Geometry check sheet. Reference: the model listing, model coordinates, mm. Face numbers are marked on the shaded views. Give positions to 0.01 mm unless a question says otherwise; leave off trailing zeros. Loops run counter-clockwise (first coordinate to the right, second up) from the corner with the lowest first, then second, coordinate; pieces in that order, holes last.
```python
from build123d import *

# Parameters (mm, degrees)
SKETCH_1_W               = 54.5
SKETCH_1_H               = 22.1
SKETCH_1_R               = 2.25
EXTRUDE_1_DEPTH          = 17
SKETCH_2_W               = 7.6
SKETCH_2_H               = 22.1
CUT_EXTRUDE_1_DEPTH      = 7.2
SKETCH_3_W               = 7.6
SKETCH_3_H               = 3.3
CUT_EXTRUDE_2_DEPTH      = 2.1
MIRROR_2_COPY_1_SKETCH_W = 7.6
MIRROR_2_COPY_1_SKETCH_H = 3.3
MIRROR_2_COPY_1_DEPTH    = 2.1
SKETCH_4_R               = 1.75
CUT_EXTRUDE_3_DEPTH      = 5


with BuildPart() as part:
    # ｽｹｯﾁ1 → ﾎﾞｽ - 押し出し1 (new body)
    with BuildSketch(Plane(origin=(0, 0, 0), x_dir=(1, 0, 0), z_dir=(0, 1, 0))):
        Rectangle(SKETCH_1_W, SKETCH_1_H)
        with Locations(Location((-22, 0, 0), (0, 0, 270))):
            Circle(SKETCH_1_R, mode=Mode.SUBTRACT)
        with Locations(Location((22, 0, 0), (0, 0, 90))):
            Circle(SKETCH_1_R, mode=Mode.SUBTRACT)
    extrude(amount=EXTRUDE_1_DEPTH)

    # ｽｹｯﾁ2 → ｶｯﾄ - 押し出し1 (cut)
    with BuildSketch(Plane(origin=(0, 17, 0), x_dir=(1, 0, 0), z_dir=(0, 1, 0))):
        with Locations((13.5, 0)):
            Rectangle(SKETCH_2_W, SKETCH_2_H)
        with Locations((-13.5, 0)):
            Rectangle(SKETCH_2_W, SKETCH_2_H)
        with Locations((-4.5, 0)):
            Rectangle(SKETCH_2_W, SKETCH_2_H)
        with Locations((4.5, 0)):
            Rectangle(SKETCH_2_W, SKETCH_2_H)
    extrude(amount=-CUT_EXTRUDE_1_DEPTH, mode=Mode.SUBTRACT)

    # ｽｹｯﾁ3 → ｶｯﾄ - 押し出し2 (cut)
    with BuildSketch(Plane(origin=(0, 9.8, 0), x_dir=(1, 0, 0), z_dir=(0, 1, 0))):
        with Locations((4.5, 9.4)):
            Rectangle(SKETCH_3_W, SKETCH_3_H)
        with Locations((13.5, 9.4)):
            Rectangle(SKETCH_3_W, SKETCH_3_H)
    cut_extrude_2 = extrude(amount=-CUT_EXTRUDE_2_DEPTH, mode=Mode.SUBTRACT)

    # ﾐﾗｰ1: ｶｯﾄ - 押し出し2 across plane
    add(cut_extrude_2.mirror(Plane(origin=(0, 0, 0), x_dir=(0, 0, 1), z_dir=(1, 0, 0))), mode=Mode.SUBTRACT)

    # ﾐﾗｰ2: ｶｯﾄ - 押し出し2 across plane
    add(cut_extrude_2.mirror(Plane.XY), mode=Mode.SUBTRACT)

    # ﾐﾗｰ2 copy 1 sketch → ﾐﾗｰ2 copy 1 (cut)
    with BuildSketch(Plane(origin=(0, 9.8, 0), x_dir=(-1, 0, 0), z_dir=(0, 1, 0))):
        with Locations((4.5, 9.4)):
            Rectangle(MIRROR_2_COPY_1_SKETCH_W, MIRROR_2_COPY_1_SKETCH_H)
        with Locations((13.5, 9.4)):
            Rectangle(MIRROR_2_COPY_1_SKETCH_W, MIRROR_2_COPY_1_SKETCH_H)
    extrude(amount=-MIRROR_2_COPY_1_DEPTH, mode=Mode.SUBTRACT)

    # ｽｹｯﾁ4 → ｶｯﾄ - 押し出し3 (cut)
    with BuildSketch(Plane(origin=(0, 9.8, 0), x_dir=(1, 0, 0), z_dir=(0, 1, 0))):
        with Locations(Location((13.5, 4, 0), (0, 0, 270))):
            Circle(SKETCH_4_R)
        with Locations(Location((4.5, 4, 0), (0, 0, 270))):
            Circle(SKETCH_4_R)
        with Locations(Location((-4.5, 4, 0), (0, 0, 270))):
            Circle(SKETCH_4_R)
        with Locations(Location((-13.5, 4, 0), (0, 0, 270))):
            Circle(SKETCH_4_R)
        with Locations(Location((13.5, -4, 0), (0, 0, 90))):
            Circle(SKETCH_4_R)
        with Locations(Location((4.5, -4, 0), (0, 0, 90))):
            Circle(SKETCH_4_R)
        with Locations(Location((-4.5, -4, 0), (0, 0, 90))):
            Circle(SKETCH_4_R)
        with Locations(Location((-13.5, -4, 0), (0, 0, 90))):
            Circle(SKETCH_4_R)
    extrude(amount=-CUT_EXTRUDE_3_DEPTH, mode=Mode.SUBTRACT)


solid = part.part
```
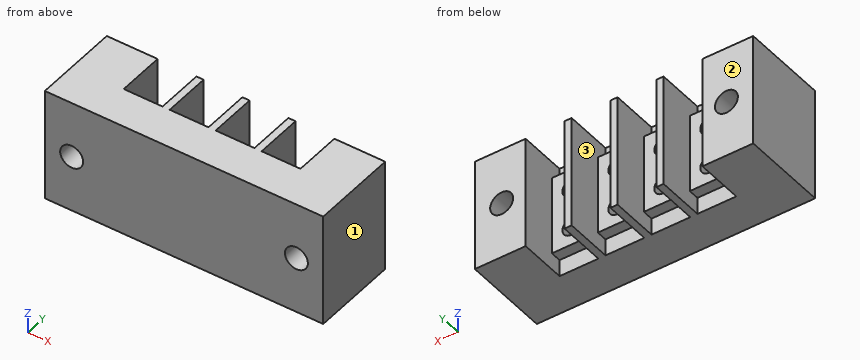
1) Sectioned sample at B-B on x = -22. Enter the section's corners in (y, z), plus the area to 3 significant figures.
2) Sectioned sample at C-C on z = 0. Enter the section's corners in (x, y).
3) Depth check by flat-ended pin: P1, Ø1, axis at x = -5.5, z = 4.5, coming from the +Y side; P2, Ø1, axis at x = -3, z = 10, coming from the +Y side; P3, Ø2.5, axis at x = 15, z = 2, coming from the +Y side. Enter the tip coordinate at first touch or a pass-through.
4) Mould release check, pull along X, two halves, no side actions. Record for the marked faces 1, 2 and 3: +X half, -X half, draft (parallel to the pull), parting line (faces both ways), or undercut.
5) Sectioned sample at A-A on y = 14.5. Enter the section's corners in (x, z), plus the area to 3 significant figures.
6) Scan lines: line 1 along X through (y, z) = (7.45, 4); line 2 along X through (y, z) = (8.5, 0); line 3 along X through (y, z) = (12.25, 9). Record each from-to range of solid material in increasing order.
7) Sectioned sample at D-D on x = -13.5. Enter the section's corners in (y, z), plus the area to 3 significant figures.
Determined:
1. outline: (0, -11.05) - (17, -11.05) - (17, -2.25) - (0, -2.25) - close; (0, 2.25) - (17, 2.25) - (17, 11.05) - (0, 11.05) - close
1. area: 299 mm2
2. outline: (-27.25, 0) - (-24.25, 0) - (-24.25, 17) - (-27.25, 17) - close; (-19.75, 0) - (19.75, 0) - (19.75, 17) - (17.3, 17) - (17.3, 9.8) - (9.7, 9.8) - (9.7, 17) - (8.3, 17) - (8.3, 9.8) - (0.7, 9.8) - (0.7, 17) - (-0.7, 17) - (-0.7, 9.8) - (-8.3, 9.8) - (-8.3, 17) - (-9.7, 17) - (-9.7, 9.8) - (-17.3, 9.8) - (-17.3, 17) - (-19.75, 17) - close; (24.25, 0) - (27.25, 0) - (27.25, 17) - (24.25, 17) - close
3. P1: stops at y = 4.8
3. P2: stops at y = 7.7
3. P3: stops at y = 9.8
4. face 1: +X half
4. face 2: draft
4. face 3: undercut
5. outline: (-27.25, -11.05) - (-17.3, -11.05) - (-17.3, 11.05) - (-27.25, 11.05) - close; (-9.7, -11.05) - (-8.3, -11.05) - (-8.3, 11.05) - (-9.7, 11.05) - close; (-0.7, -11.05) - (0.7, -11.05) - (0.7, 11.05) - (-0.7, 11.05) - close; (8.3, -11.05) - (9.7, -11.05) - (9.7, 11.05) - (8.3, 11.05) - close; (17.3, -11.05) - (27.25, -11.05) - (27.25, 11.05) - (17.3, 11.05) - close; hole circle Ø4.5 at (-22, 0); hole circle Ø4.5 at (22, 0)
5. area: 501 mm2
6. line 1: x = -27.25 to -15.25, -11.75 to -6.25, -2.75 to 2.75, 6.25 to 11.75, 15.25 to 27.25
6. line 2: x = -27.25 to -24.25, -19.75 to 19.75, 24.25 to 27.25
6. line 3: x = -27.25 to -17.3, -9.7 to -8.3, -0.7 to 0.7, 8.3 to 9.7, 17.3 to 27.25
7. outline: (0, -11.05) - (7.7, -11.05) - (7.7, -7.75) - (9.8, -7.75) - (9.8, -5.75) - (4.8, -5.75) - (4.8, -2.25) - (9.8, -2.25) - (9.8, 2.25) - (4.8, 2.25) - (4.8, 5.75) - (9.8, 5.75) - (9.8, 7.75) - (7.7, 7.75) - (7.7, 11.05) - (0, 11.05) - close
7. area: 168 mm2
